Could you check a few things on this drawing? It's one solid part, dimensions in mm from its lowest x, y, z. A direction names the side the tool comes from. Coordinates: 2 decimals unless noted, no trailing zeros. Order: outer loops, then holes, each group sorted by start corner. A loop starts at its lowest first (then second) coordinate and runs counter-clockwise, first axis right, second up. Notation, with made-up numbers: (8, 79) - (35, 79) arc R23 ccw to (35, 112) - close; hole circle Ø1 at (54.25, 66). An arc over 180 degrees is marked (long way). Answer in a Markdown table with one row per item. Add a question column.
Item 1: Will this pin go through, and if not, where does the flat tip stop? pin 1 Ø2 at (x, y) = (6.5, 8.5) entering from +Z.
Item 2: I want a section at B-B (z = 2.85). Please give me the cut outline in (x, y).
Item 3: I want a section at A-A (y = 3.75). Please give me the cut outline in (x, z).
Item 4: On a 3-axis mill with a long thin cutter (end or side, diameter ignored), from which of +Z, -Z, +X, -X, +Y, -Y can I reach the whole of each face in a straight line? I mean the marked faces 1, 2 and 3. Say none if no direction works.
Item 5: I want a section at C-C (x = 6.75). Please give me the cut outline in (y, z).
Item 6: I want a section at D-D (x = 2). Please give me the cut outline in (y, z), plus the area to 3 significant figures.
Item 7: If I drill on line 1 along Y through (x, z) = (7.75, 2.7); line 2 along Y through (x, z) = (0.75, 1.2); line 3 along X through (y, z) = (3, 1.8), over which ranges is the centre line in solid material (lowest first)? Write a range as from..to.
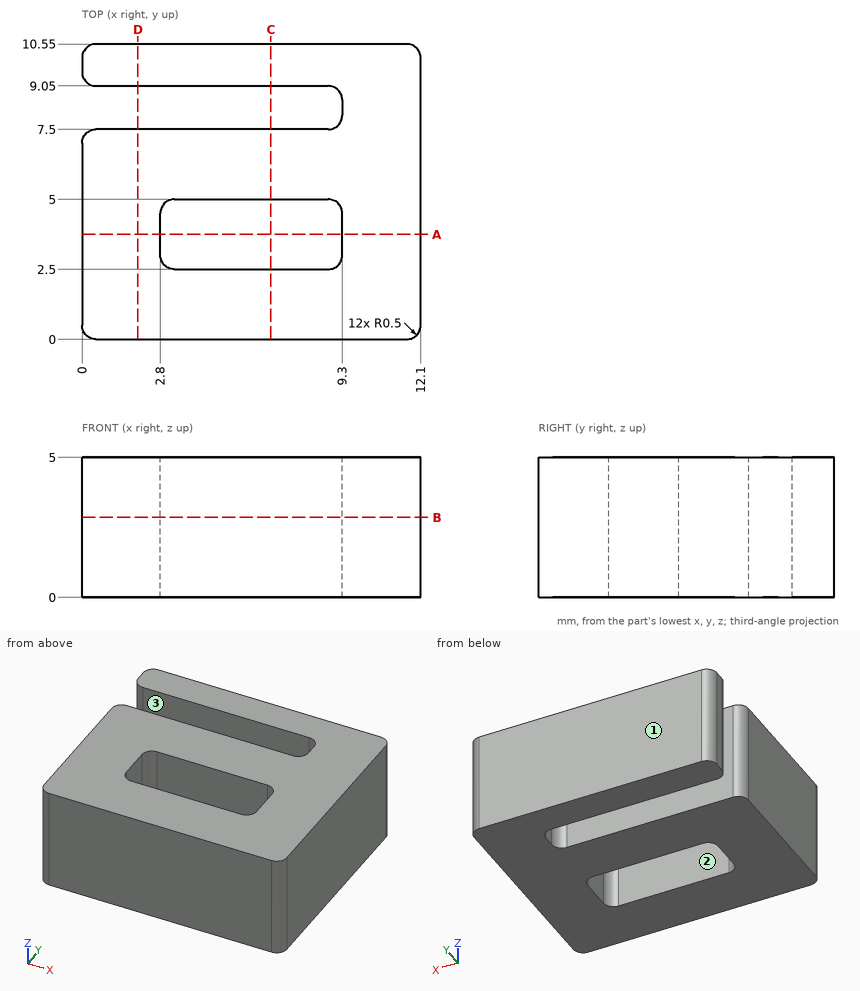
Values follow:
| question | item | result |
|---|---|---|
| 1 | pin 1 | stops at z = 5 |
| 2 | outline | (0, 0.5) arc R0.5 ccw to (0.5, 0) - (11.6, 0) arc R0.5 ccw to (12.1, 0.5) - (12.1, 10.05) arc R0.5 ccw to (11.6, 10.55) - (0.5, 10.55) arc R0.5 ccw to (0, 10.05) - (0, 9.55) arc R0.5 ccw to (0.5, 9.05) - (8.8, 9.05) arc R0.5 cw to (9.3, 8.55) - (9.3, 8) arc R0.5 cw to (8.8, 7.5) - (0.5, 7.5) arc R0.5 ccw to (0, 7) - close; hole (2.8, 3) arc R0.5 ccw to (3.3, 2.5) - (8.8, 2.5) arc R0.5 ccw to (9.3, 3) - (9.3, 4.5) arc R0.5 ccw to (8.8, 5) - (3.3, 5) arc R0.5 ccw to (2.8, 4.5) - close |
| 3 | outline | (0, 0) - (2.8, 0) - (2.8, 5) - (0, 5) - close; (9.3, 0) - (12.1, 0) - (12.1, 5) - (9.3, 5) - close |
| 4 | face 1 | +Z, -Z, +X, -X, +Y |
| 4 | face 2 | +Z, -Z |
| 4 | face 3 | +Z, -Z, -X |
| 5 | outline | (0, 0) - (2.5, 0) - (2.5, 5) - (0, 5) - close; (5, 0) - (7.5, 0) - (7.5, 5) - (5, 5) - close; (9.05, 0) - (10.55, 0) - (10.55, 5) - (9.05, 5) - close |
| 6 | outline | (0, 0) - (7.5, 0) - (7.5, 5) - (0, 5) - close; (9.05, 0) - (10.55, 0) - (10.55, 5) - (9.05, 5) - close |
| 6 | area | 45.0 mm^2 |
| 7 | line 1 | y = 0..2.5, 5..7.5, 9.05..10.55 |
| 7 | line 2 | y = 0..7.5, 9.05..10.55 |
| 7 | line 3 | x = 0..2.8, 9.3..12.1 |
